Can you work these out from the model? Positions are in its coordinate system, mm. Coordinates: 2 decimals unless noted, no trailing zeros. Loops run counter-clockwise (first coordinate to the right, second up) from the corner with the lowest first, then second, coordinate; pieces in that order, holes last. Notation, with made-up numbers: M 25,-20 L 50,-20 A15 ccw 50,-5 Z; hole C 4,75 d10. An arc over 180 degrees is marked long. Answer as a JSON object with one key per item and string values. Group by question number.
Item 1: Suppose I cut it at A-A (x = 47). Write out the boundary of the cut face in (y, z), then the cut area to 3 significant figures.
Item 2: If I drill on line 1 (X direction, y = 1.1, z = 31); line 2 (X direction, y = 1, z = -15); line 3 (Z direction, x = -13.5, y = 2.8), over which ranges is the centre line in solid material (lowest first)?
Item 3: Suppose I cut it at B-B (z = -31). Write out the boundary of the cut face in (x, y).
Item 4: We'd pull the mould along X, two halves only. Please class faces 1 (the cylindrical face through (48.81, 1.48, -13.84)), 2 (the flat face through (17, 1, -35)), 3 (the flat face through (-18, 1, 0)): +X half, -X half, draft (parallel to the pull), parting line (faces both ways), or undercut.
Item 5: I'm going to push a flat-ended pin straight in: pin 1 Ø3.5 at (x, z) = (-15, -31) entering from +Y. Where does the tip first touch, or does it pass through?
Item 6: Suppose I cut it at C-C (y = 1.4). Write out the boundary of the cut face in (x, z), then the cut area to 3 significant figures.
Item 7: Suppose I cut it at D-D (x = -15). Write out the boundary of the cut face in (y, z).
```python
from build123d import *

# Parameters (mm, degrees)
SKETCH1_R           = 2.15
BOSS_EXTRUDE1_DEPTH = 3


with BuildPart() as part:
    # Sketch1 → Boss-Extrude1 (new body)
    with BuildSketch(Plane(origin=(0, 0, 0), x_dir=(1, 0, 0), z_dir=(0, 1, 0))):
        Polygon((18, 35), (51, 35), (51, -35), (18, -35), (-18, -35), (-18, 35), align=None)
        with Locations(Location((15, 31, 0), (0, 0, 270))):
            Circle(SKETCH1_R, mode=Mode.SUBTRACT)
        with Locations(Location((-15, 31, 0), (0, 0, 270))):
            Circle(SKETCH1_R, mode=Mode.SUBTRACT)
        with Locations(Location((-15, -31, 0), (0, 0, 270))):
            Circle(SKETCH1_R, mode=Mode.SUBTRACT)
        with Locations(Location((15, -31, 0), (0, 0, 270))):
            Circle(SKETCH1_R, mode=Mode.SUBTRACT)
        with Locations(Location((47, 15, 0), (0, 0, 270))):
            Circle(SKETCH1_R, mode=Mode.SUBTRACT)
    extrude(amount=BOSS_EXTRUDE1_DEPTH)


solid = part.part
```
From the geometry:
{
 "1": {"outline": "M 0,-35 L 3,-35 L 3,-17.15 L 0,-17.15 Z; M 0,-12.85 L 3,-12.85 L 3,35 L 0,35 Z", "area": "197 mm2"},
 "2": {"line 1": "-18 to -17.15, -12.85 to 12.85, 17.15 to 51", "line 2": "-18 to 44.85, 49.15 to 51", "line 3": "-35 to -32.54, -29.46 to 29.46, 32.54 to 35"},
 "3": {"outline": "M -18,0 L -17.15,0 L -17.15,3 L -18,3 Z; M -12.85,0 L 12.85,0 L 12.85,3 L -12.85,3 Z; M 17.15,0 L 51,0 L 51,3 L 17.15,3 Z"},
 "4": {"face 1": "undercut", "face 2": "draft", "face 3": "-X half"},
 "5": {"pin 1": "through"},
 "6": {"outline": "M -18,-35 L 51,-35 L 51,35 L -18,35 Z; hole C -15,-31 d4.3; hole C -15,31 d4.3; hole C 15,-31 d4.3; hole C 15,31 d4.3; hole C 47,-15 d4.3", "area": "4,760 mm2"},
 "7": {"outline": "M 0,-35 L 3,-35 L 3,-33.15 L 0,-33.15 Z; M 0,-28.85 L 3,-28.85 L 3,28.85 L 0,28.85 Z; M 0,33.15 L 3,33.15 L 3,35 L 0,35 Z"}
}
